```python
from build123d import *

# Parameters (mm, degrees)
F1_DEPTH = 6.2


with BuildPart() as f1:
    # F0 (on Front) → F1 (new body)
    with BuildSketch(Plane.XZ):
        with BuildLine():
            ThreePointArc((-8, 3), (-11, 0), (-8, -3))
            ThreePointArc((-8, -3), (-5.8786796564, -2.1213203436), (-5, 0))
            ThreePointArc((-5, 0), (-5.8786796564, 2.1213203436), (-8, 3))
        make_face()
        with BuildLine():
            Line((-8, -3), (8, -3))
            ThreePointArc((8, -3), (5, 0), (8, 3))
            Line((8, 3), (-8, 3))
            ThreePointArc((-8, 3), (-5.8786796564, 2.1213203436), (-5, 0))
            ThreePointArc((-5, 0), (-5.8786796564, -2.1213203436), (-8, -3))
        make_face()
        with BuildLine():
            ThreePointArc((8, 3), (5, 0), (8, -3))
            ThreePointArc((8, -3), (10.1213203436, -2.1213203436), (11, 0))
            ThreePointArc((11, 0), (10.1213203436, 2.1213203436), (8, 3))
        make_face()
    extrude(amount=F1_DEPTH)


solid = f1.part
```
Geometry: final body of the model. Coordinates: model frame, mm. Round coordinates to 2 decimals unless told otherwise and drop trailing zeros. Order: outer loops, then holes, each group sorted by start corner. A loop starts at its lowest first (then second) coordinate and runs counter-clockwise, first axis right, second up. Notation, with made-up numbers: (11.5, 50) -> (35.5, 50) arc R17 cw to (35.5, 74) -> close; hole circle Ø5 at (-25.75, 35.25). An arc over 180 degrees is marked (long way). Use one line per item in the form item = value.
(1) Section B-B on z = -2.5. Return loops of the section in (x, y), and give its area (3 significant figures).
Results list:
outline = (-9.66, -6.2) -> (9.66, -6.2) -> (9.66, 0) -> (-9.66, 0) -> close
area = 120 mm^2
(2) Section A-A on y = -2. Return loops of the section in (x, z), and give its area (3 significant figures).
Results list:
outline = (-8, -3) -> (8, -3) arc R3 ccw to (8, 3) -> (-8, 3) arc R3 ccw to start
area = 124 mm^2
(3) Ray query, probe 1 along X at (y, z) = (-1, 2); probe 2 along X at (y, z) = (-4.5, -1.5); probe 3 along Z at (x, y) = (9.25, -2.75). Return the intervals inside material, ascending. Write a range as [from, to].
Results list:
probe_1 = [-10.24, 10.24]
probe_2 = [-10.6, 10.6]
probe_3 = [-2.73, 2.73]
(4) Section C-C on z = -1.5. Return loops of the section in (x, y).
Results list:
outline = (-10.6, -6.2) -> (10.6, -6.2) -> (10.6, 0) -> (-10.6, 0) -> close
